Could you check a few things on this drawing? It's one solid part, dimensions in mm from its lowest x, y, z. A direction names the side the tool comes from. Give positions to 0.01 mm unless a question says otherwise; leave off trailing zeros. Loops run counter-clockwise (first coordinate to the right, second up) from the corner with the lowest first, then second, coordinate; pieces in that order, holes last. Notation, with made-up numbers: M 46,-18 L 75,-18 A32 ccw 75,15 Z; hole C 60.25,66 d10. An arc over 180 degrees is marked long. One line per item, written item: value. Start each with the question number.
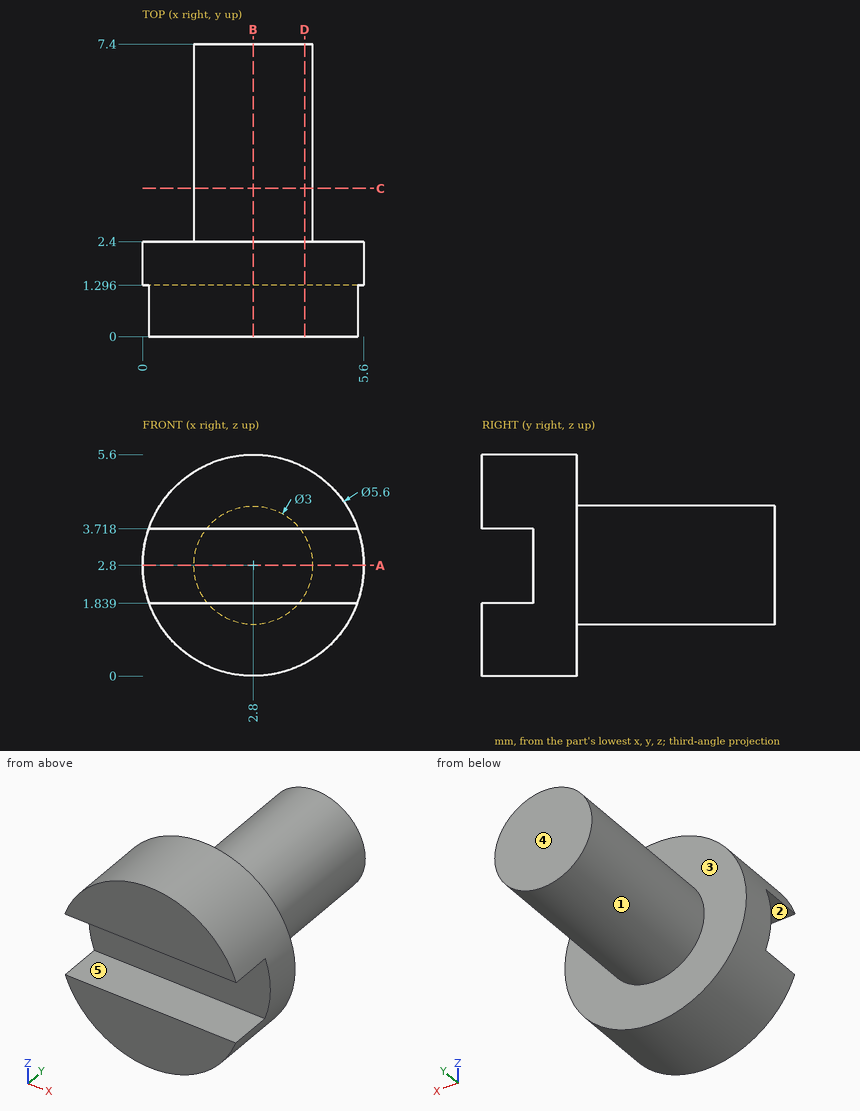
Q1. Which directions (+Z, -Z, +X, -X, +Y, -Y) give clear straight access to the entire face, cutting with the end or side of a thin tool? Please do the marked faces 4 and 5.
Q2. If we section it at D-D, the plane x = 4.1: Write out the boundary of the cut face in (y, z).
Q3. If we mould it in two halves opening along Z, with no side actions, what happens to the marked faces 1, 2 and 3? For each: released by +Z, released by -Z, zero draft, split by the parting line, or undercut.
Q4. I need wall thicknesses on line 1 along Y through (x, z) = (3.4, 3.15); line 2 along Y through (x, z) = (4.1, 0.75); line 3 along Z through (x, y) = (4.05, 0.75) (1 decimal). Which ranges of each line are inside material? Lowest first, please.
Q5. For P1, Ø1.5, axis at x = 3.5, y = 5, coming from the -Z side; P2, Ø3, axis at x = 4.5, z = 4.5, coming from the +Y side; P3, Ø1, axis at x = 2, z = 5, coming from the +Y side, each with a flat end and sliding along its axis, tell me the tip position at first contact or that it passes through.
Q6. If we section it at C-C, the plane y = 3.75: Write out the boundary of the cut face in (x, z).
Q7. If we section it at A-A, the plane z = 2.8: Write out the boundary of the cut face in (x, y).
Q8. If we section it at B-B, the plane x = 2.8: Write out the boundary of the cut face in (y, z).
Response:
1. face 4: +Z, -Z, +X, -X, +Y
1. face 5: +X, -X, -Y
2. outline: M 0,0.32 L 2.4,0.32 L 2.4,2.05 L 7.4,2.05 L 7.4,3.55 L 2.4,3.55 L 2.4,5.28 L 0,5.28 L 0,3.72 L 1.3,3.72 L 1.3,1.84 L 0,1.84 Z
3. face 1: split by the parting line
3. face 2: undercut
3. face 3: zero draft
4. line 1: 1.3 to 7.4
4. line 2: 0 to 2.4
4. line 3: 0.3 to 1.8, 3.7 to 5.3
5. P1: z = 1.3
5. P2: y = 7.4
5. P3: y = 2.4
6. outline: C 2.8,2.8 d3
7. outline: M 0,1.3 L 5.6,1.3 L 5.6,2.4 L 4.3,2.4 L 4.3,7.4 L 1.3,7.4 L 1.3,2.4 L 0,2.4 Z
8. outline: M 0,0 L 2.4,0 L 2.4,1.3 L 7.4,1.3 L 7.4,4.3 L 2.4,4.3 L 2.4,5.6 L 0,5.6 L 0,3.72 L 1.3,3.72 L 1.3,1.84 L 0,1.84 Z
